```python
from build123d import *

# Parameters (mm, degrees)
BOSS_EXTRUDE1_DEPTH     = 4.85
CUT_EXTRUDE1_DEPTH      = 44.672701752
CUT_EXTRUDE1_DEPTH_BACK = 44.672701752
SKETCH3_R               = 1.2
CUT_EXTRUDE2_DEPTH      = 4


with BuildPart() as part:
    # Sketch1 → Boss-Extrude1 (new, symmetric)
    with BuildSketch(Plane.XY):
        with BuildLine():
            Line((-15.15, 19.9), (15.15, 19.9))
            Line((15.15, 19.9), (30, -6.9))
            ThreePointArc((30, -6.9), (31.992906647, -7.162371138), (33.85, -7.931604391))
            Line((33.85, -7.931604391), (32.5, -10.269872981))
            ThreePointArc((32.5, -10.269872981), (25.301536896, -16.310100717), (34.698463104, -16.310100717))
            Line((34.698463104, -16.310100717), (37.23563318, -17.233555104))
            ThreePointArc((37.23563318, -17.233555104), (28.662909032, -22.183019698), (22.3, -14.6))
            Line((22.3, -14.6), (8.25, 14.6))
            Line((8.25, 14.6), (-8.25, 14.6))
            Line((-8.25, 14.6), (-22.3, -14.6))
            ThreePointArc((-22.3, -14.6), (-28.662909032, -22.183019698), (-37.23563318, -17.233555104))
            Line((-37.23563318, -17.233555104), (-34.698463104, -16.310100717))
            ThreePointArc((-34.698463104, -16.310100717), (-25.301536896, -16.310100717), (-32.5, -10.269872981))
            Line((-32.5, -10.269872981), (-33.85, -7.931604391))
            ThreePointArc((-33.85, -7.931604391), (-31.992906647, -7.162371138), (-30, -6.9))
            Line((-30, -6.9), (-15.15, 19.9))
        make_face()
    extrude(amount=BOSS_EXTRUDE1_DEPTH, both=True)

    # Sketch2 → Cut-Extrude1 (cut, two sides: drawn at the far end of the back side and taken through both)
    with BuildSketch(Plane.XY.offset(-CUT_EXTRUDE1_DEPTH_BACK)):
        with BuildLine():
            Line((-26.925180599, -7.540574694), (-16.546196528, 11.190521138))
            ThreePointArc((-16.546196528, 11.190521138), (-14.545175942, 11.795919776), (-13.88248318, 9.813136581))
            Line((-13.88248318, 9.813136581), (-23.582107554, -10.345513363))
            ThreePointArc((-23.582107554, -10.345513363), (-25.050776345, -8.701255624), (-26.925180599, -7.540574694))
        make_face()
        with BuildLine():
            Line((13.88248318, 9.813136581), (23.582107554, -10.345513363))
            ThreePointArc((23.582107554, -10.345513363), (25.050776345, -8.701255624), (26.925180599, -7.540574694))
            Line((26.925180599, -7.540574694), (16.546196528, 11.190521138))
            ThreePointArc((16.546196528, 11.190521138), (14.545175942, 11.795919776), (13.88248318, 9.813136581))
        make_face()
    extrude(amount=CUT_EXTRUDE1_DEPTH + CUT_EXTRUDE1_DEPTH_BACK, mode=Mode.SUBTRACT)

    # Sketch3 → Cut-Extrude2 (cut)
    with BuildSketch(Plane(origin=(0, 19.9, 0), x_dir=(1, 0, 0), z_dir=(0, 1, 0))):
        with Locations(Location((-12.475, 0, 0), (0, 0, 270))):
            Circle(SKETCH3_R)
        with Locations(Location((12.475, 0, 0), (0, 0, 270))):
            Circle(SKETCH3_R)
    extrude(amount=-CUT_EXTRUDE2_DEPTH, mode=Mode.SUBTRACT)


solid = part.part
```
CAD build for the part. Positions are in the model's coordinates, mm. A direction names the side the tool comes from. Round coordinates to 2 decimals unless told otherwise and drop trailing zeros. Order: outer loops, then holes, each group sorted by start corner. A loop starts at its lowest first (then second) coordinate and runs counter-clockwise, first axis right, second up. Notation, with made-up numbers: (-34.75, 85) -> (-8.75, 85) arc R22 ccw to (-8.75, 110) -> close; hole circle Ø7 at (21.25, 30). An arc over 180 degrees is marked (long way). Write item = value, one per line.
(1) Cut at D-D (x = -10). Write the cut outline in (y, z).
Answers follow:
outline = (10.96, -4.85) -> (19.9, -4.85) -> (19.9, 4.85) -> (10.96, 4.85) -> close
(2) 3-axis set-ups, long thin cutter, end or side, ignore diameter. For faces 1 (the flat face through (33.184, -9.084, 0.068)), 2 (the flat face through (-18.664, -0.125, -0.068)), 3 (the cylindrical face through (11.304, 17.928, -0.26)): which of +Z, -Z, +X, -X, +Y, -Y reach the whole face in a straight line?
Answers follow:
face_1 = +Z, -Z, +X
face_2 = +Z, -Z
face_3 = +Y
(3) Drill centre lines: L1, parallel to Y at x = 30, z = 3.25; L2, parallel to X at y = -14.6, z = -2.25; L3, parallel to X at y = -1.5, z = -3. Where is each one in solid material? Low to high.
Answers follow:
L1 = -22.3 to -19.6, -9.6 to -6.9
L2 = -25 to -22.3, 22.3 to 25
L3 = -27.01 to -23.58, -19.33 to -16, 16 to 19.33, 23.58 to 27.01
(4) Flat gauge pins, fed straight in: P1, Ø1.5, axis at y = -5.5, z = -1, coming from the -X side; P2, Ø1.2, axis at x = 12, z = 0, coming from the +Y side; P3, Ø1.9, axis at x = 12.475, z = 0, coming from the -Y side. Where does each tip first touch, or does it go through?
Answers follow:
P1 = -29.64
P2 = 15.9
P3 = 3.84
(5) Cut at B-B (y = 2). Write the cut outline in (x, z).
Answers follow:
outline = (-25.07, -4.85) -> (-21.64, -4.85) -> (-21.64, 4.85) -> (-25.07, 4.85) -> close; (-17.64, -4.85) -> (-14.31, -4.85) -> (-14.31, 4.85) -> (-17.64, 4.85) -> close; (14.31, -4.85) -> (17.64, -4.85) -> (17.64, 4.85) -> (14.31, 4.85) -> close; (21.64, -4.85) -> (25.07, -4.85) -> (25.07, 4.85) -> (21.64, 4.85) -> close
(6) Cut at A-A (z = -2). Write the cut outline in (x, y), plus the area to 3 significant figures.
Answers follow:
outline = (-37.24, -17.23) arc R7.7 ccw to (-22.3, -14.6) -> (-8.25, 14.6) -> (8.25, 14.6) -> (22.3, -14.6) arc R7.7 ccw to (37.24, -17.23) -> (34.7, -16.31) arc R5 cw (long way) to (32.5, -10.27) -> (33.85, -7.93) arc R7.7 ccw to (30, -6.9) -> (15.15, 19.9) -> (-15.15, 19.9) -> (-30, -6.9) arc R7.7 ccw to (-33.85, -7.93) -> (-32.5, -10.27) arc R5 cw (long way) to (-34.7, -16.31) -> close; hole (-26.93, -7.54) arc R7.7 cw to (-23.58, -10.35) -> (-13.88, 9.81) arc R1.5 ccw to (-16.55, 11.19) -> close; hole (13.88, 9.81) -> (23.58, -10.35) arc R7.7 cw to (26.93, -7.54) -> (16.55, 11.19) arc R1.5 ccw to start
area = 691 mm²
(7) Cut at C-C (x = 7). Write the cut outline in (y, z), plus the area to 3 significant figures.
Answers follow:
outline = (14.6, -4.85) -> (19.9, -4.85) -> (19.9, 4.85) -> (14.6, 4.85) -> close
area = 51.4 mm²
(8) Pull direction Y, two halves, no side cores. Call faces 4 (the cylindrical face through (14.57, 11.81, -0.07)), 5 (the flat face through (-15.18, 0.2, 0.07)), 6 (the flat face through (0, 19.9, 0)): +Y half, -Y half, draft (parallel to the pull), parting line (faces both ways), or undercut.
Answers follow:
face_4 = undercut
face_5 = -Y half
face_6 = +Y half
